CAD build for the part. Positions are in the model's coordinates, mm. A direction names the side the tool comes from. Give positions to 0.01 mm unless a question says otherwise; leave off trailing zeros. Write each loop counter-clockwise with the first axis right and the second up, starting at its lowest first coordinate (ties: lowest second). Pieces come first, ordered by that corner, then holes. Notation, with made-up numbers: (61.25, 32.25) -> (81.25, 32.25) arc R26 cw to (81.25, 51.25) -> close; hole circle Ø3 at (61.5, 70). An arc over 180 degrees is marked (long way). Answer in a Markdown table with one row per item. Add a question column.
```python
from build123d import *

# Parameters (mm, degrees)
BOSS_EXTRUDE1_DEPTH = 140
SKETCH2_R           = 18.75
CUT_EXTRUDE1_DEPTH  = 5.16


with BuildPart() as part:
    # Sketch1 → Boss-Extrude1 (new body)
    with BuildSketch(Plane(origin=(0, 0, 0), x_dir=(0, 0, -1), z_dir=(1, 0, 0))):
        Polygon((-4.84, 12.650615569), (-10, 12.650615569), (-10, -12.650615569), (-4.84, -12.650615569), (-4.84, -19.34), (10, -19.34), (10, 19.34), (-4.84, 19.34), align=None)
    extrude(amount=BOSS_EXTRUDE1_DEPTH)

    # Sketch2 → Cut-Extrude1 (cut)
    with BuildSketch(Plane.XY.offset(10)):
        with Locations((70, 0)):
            Circle(SKETCH2_R)
    extrude(amount=-CUT_EXTRUDE1_DEPTH, mode=Mode.SUBTRACT)


solid = part.part
```
Item 1: Slice it at D-D, the plane x = 78. List the corners of the cut face in (y, z), then the cut area to 3 significant figures.
Item 2: Mould opens along Y. For faces 6 (the face through (88.75, -0.19, 7.46)), 7 (the face through (69, 19.34, -3)), 8 (the face through (28, -12.651, 7)), 9 (the face through (69, 0, -10)) say: released by +Y, released by -Y, zero draft, split by the parting line, or undercut.
Item 3: Slice it at B-B, the plane x = 9. List the corners of the cut face in (y, z), then the cut area to 3 significant figures.
Item 4: Which spindle directions (+Z, -Z, +X, -X, +Y, -Y) get a long thin tool onto all of the face, cutting with end or side? Do faces 1 (the face through (112, 0, 10)), 2 (the face through (112, -12.651, 7)), 3 (the face through (0, 0, 0)), 4 (the face through (28, 12.651, 7)), 5 (the face through (51.25, 0.19, 7.46)). Say none if no direction does.
Item 5: Probe L1, parallel to Z at x = 109, y = 13.5; L2, parallel to X at y = 6.5, z = 6.5; L3, parallel to X at y = 1.5, z = 5.75. List the from-to ranges inside material, lowest first. Write a range as from..to.
Item 6: Slice it at C-C, the plane y = -7. List the corners of the cut face in (x, z).
Item 7: Drop flat-ended pins along their axis: pin 1 Ø1.5 at (x, z) = (112.5, 8.5) entering from -Y; pin 2 Ø11.5 at (x, y) = (63, 5.5) entering from +Z; pin 3 Ø2.5 at (x, z) = (16.5, 7) entering from +Y. Give the stop position or say it passes through.
Item 8: Slice it at A-A, the plane z = 8.5. List the corners of the cut face in (x, y).
Answer key:
| question | item | result |
|---|---|---|
| 1 | outline | (-19.34, -10) -> (19.34, -10) -> (19.34, 4.84) -> (-19.34, 4.84) -> close |
| 1 | area | 574 mm² |
| 2 | face 6 | undercut |
| 2 | face 7 | released by +Y |
| 2 | face 8 | released by -Y |
| 2 | face 9 | zero draft |
| 3 | outline | (-19.34, -10) -> (19.34, -10) -> (19.34, 4.84) -> (12.65, 4.84) -> (12.65, 10) -> (-12.65, 10) -> (-12.65, 4.84) -> (-19.34, 4.84) -> close |
| 3 | area | 705 mm² |
| 4 | face 1 | +Z, +X, -X, +Y, -Y |
| 4 | face 2 | +Z, +X, -X, -Y |
| 4 | face 3 | +Z, -Z, -X, +Y, -Y |
| 4 | face 4 | +Z, +X, -X, +Y |
| 4 | face 5 | +Z |
| 5 | L1 | z = -10..4.84 |
| 5 | L2 | x = 0..52.41, 87.59..140 |
| 5 | L3 | x = 0..51.31, 88.69..140 |
| 6 | outline | (0, -10) -> (140, -10) -> (140, 10) -> (87.39, 10) -> (87.39, 4.84) -> (52.61, 4.84) -> (52.61, 10) -> (0, 10) -> close |
| 7 | pin 1 | stops at y = -12.65 |
| 7 | pin 2 | stops at z = 4.84 |
| 7 | pin 3 | stops at y = 12.65 |
| 8 | outline | (0, -12.65) -> (56.16, -12.65) arc R18.75 cw to (56.16, 12.65) -> (0, 12.65) -> close; (83.84, -12.65) -> (140, -12.65) -> (140, 12.65) -> (83.84, 12.65) arc R18.75 cw to start |
